```python
from build123d import *

# Parameters (mm, degrees)
CROQUIS2_R            = 12.5
CORTAR_EXTRUIR1_DEPTH = 20
CORTAR_EXTRUIR1_TAPER = 5
CROQUIS3_R            = 5.164873121
CORTAR_EXTRUIR2_DEPTH = 79.0000001
MATRIZC2_COUNT        = 6


with BuildPart() as part:
    # Croquis1 → Revolución1 (revolve)
    with BuildSketch(Plane.XY):
        with BuildLine():
            Line((0, 0), (0, 90))
            Line((0, 90), (20, 90))
            Line((20, 90), (20, 81))
            Line((20, 81), (28, 81))
            Line((28, 81), (30, 79))
            Line((30, 79), (30, 62.9949995))
            ThreePointArc((30, 62.9949995), (30.585786438, 61.580785938), (32, 60.9949995))
            Line((32, 60.9949995), (32, 50.9949995))
            ThreePointArc((32, 50.9949995), (39.5, 33.141428429), (57.5, 26))
            Line((57.5, 26), (57.5, 22))
            Line((57.5, 22), (80, 22))
            ThreePointArc((80, 22), (85, 17), (80, 12))
            Line((80, 12), (40, 12))
            Line((40, 12), (40, 0))
            Line((40, 0), (0, 0))
        make_face()
    revolve(axis=Axis((0, 0, 0), (0, 1, 0)))

    # Croquis2 → Cortar-Extruir1 (cut)
    with BuildSketch(Plane(origin=(0, 90, 0), x_dir=(1, 0, 0), z_dir=(0, 1, 0))):
        Circle(CROQUIS2_R)
    extrude(amount=-CORTAR_EXTRUIR1_DEPTH, taper=CORTAR_EXTRUIR1_TAPER, mode=Mode.SUBTRACT)

    # Croquis3 → Cortar-Extruir2 (cut, through all)
    with BuildSketch(Plane.XZ.offset(-12)):
        with Locations((0, 70)):
            Circle(CROQUIS3_R)
    cortar_extruir2 = extrude(amount=-CORTAR_EXTRUIR2_DEPTH, mode=Mode.SUBTRACT)

    # MatrizC2: Cortar-Extruir2 ×6 about axis
    matrizc2_axis = Axis((0, 0, 0), (0, 1, 0))
    for i in range(1, MATRIZC2_COUNT):
        add(cortar_extruir2.rotate(matrizc2_axis, i * 360 / MATRIZC2_COUNT), mode=Mode.SUBTRACT)


solid = part.part
```
Check sheet for the modelled part. Datum: model origin and axes. Units: mm. A direction names the side the tool comes from. Round coordinates to 2 decimals unless told otherwise and drop trailing zeros. Order: outer loops, then holes, each group sorted by start corner. A loop starts at its lowest first (then second) coordinate and runs counter-clockwise, first axis right, second up. Notation, with made-up numbers: (49, 54.5) -> (79, 54.5) arc R30 cw to (79, 77.5) -> close; hole circle Ø11 at (78.25, -33). An arc over 180 degrees is marked (long way). One line per item, written item: value. Start each with the question number.
Q1. Gauge pin test, flat ends, axial feed: pin 1 Ø13.5 at (x, z) = (60.62, 35) entering from -Y; pin 2 Ø4 at (x, y) = (17.5, 19.5) entering from +Z; pin 3 Ø1 at (y, z) = (13, 42.5) entering from -X. Record the tip position at first contact, or that the pin passes through.
Q2. Cross-section at D-D (y = 57). Record the boundary of the cut face in (x, z).
Q3. Cross-section at B-B (y = 67). Record the boundary of the cut face in (x, z).
Q4. Thickness scan on line 1 (Z direction, x = 0, y = 16.75); line 2 (Z direction, x = 0, y = 15.25); line 3 (Y direction, x = 75, z = -7.5). Record the ranges inside material, lowest first.
Q5. Mould release check, pull along X, two halves, no side actions. Record for faces 1 (the face through (-12.465, 23.972, 56.133)), 2 (the face through (-1, 0, -1)), 3 (the face through (-0.67, 16.93, 75.12)): pulls with the +X half, pulls with the -X half, needs draft (parallel to the pull), parting line crosses it, or undercut.
Q6. Set-up check for faces 4 (the face through (-8.67, 5.92, 39.05)), 5 (the face through (-29.97, 70.89, -1.32)), 6 (the face through (-64.43, 16.93, -31.51)): record each of +Z, -Z, +X, -X, +Y, -Y from which the full face is reachable in a straight line by a thin tool's end or side.
Q7. Cross-section at A-A (z = 35). Give the number of separate pieces and of enclosed holes in the cut face, and give its area (3 significant figures).
Q8. Cross-section at C-C (y = 84.5). Record the boundary of the cut face in (x, z).
Completed:
1. pin 1: stops at y = 12
1. pin 2: stops at z = 83.34
1. pin 3: stops at x = -72.03
2. outline: circle Ø64 at (0, 0)
3. outline: circle Ø60 at (0, 0)
4. line 1: z = -84.99 to -75.16, -64.84 to 64.84, 75.16 to 84.99
4. line 2: z = -84.68 to -75.16, -64.84 to 64.84, 75.16 to 84.68
4. line 3: y = 12 to 22
5. face 1: parting line crosses it
5. face 2: needs draft
5. face 3: undercut
6. face 4: -Y
6. face 5: +Y
6. face 6: +Y, -Y
7. separate pieces: 3
7. enclosed holes: 0
7. area: 2,680 mm²
8. outline: circle Ø40 at (0, 0); hole circle Ø24.04 at (0, 0)
